Drawing for the job (mm, zero at the part's lowest x, y, z). A direction names the side the tool comes from. Coordinates: 2 decimals unless noted, no trailing zeros. Write each loop counter-clockwise with the first axis right and the second up, starting at its lowest first coordinate (ties: lowest second). Pieces come first, ordered by that corner, then holes. Notation, with made-up numbers: (22.25, 42) - (72.25, 42) arc R27 ccw to (72.25, 69) - close; hole circle Ø7 at (53, 27.5). An arc over 180 degrees is marked (long way). Write each question's results on one line, items separated by ' | '.
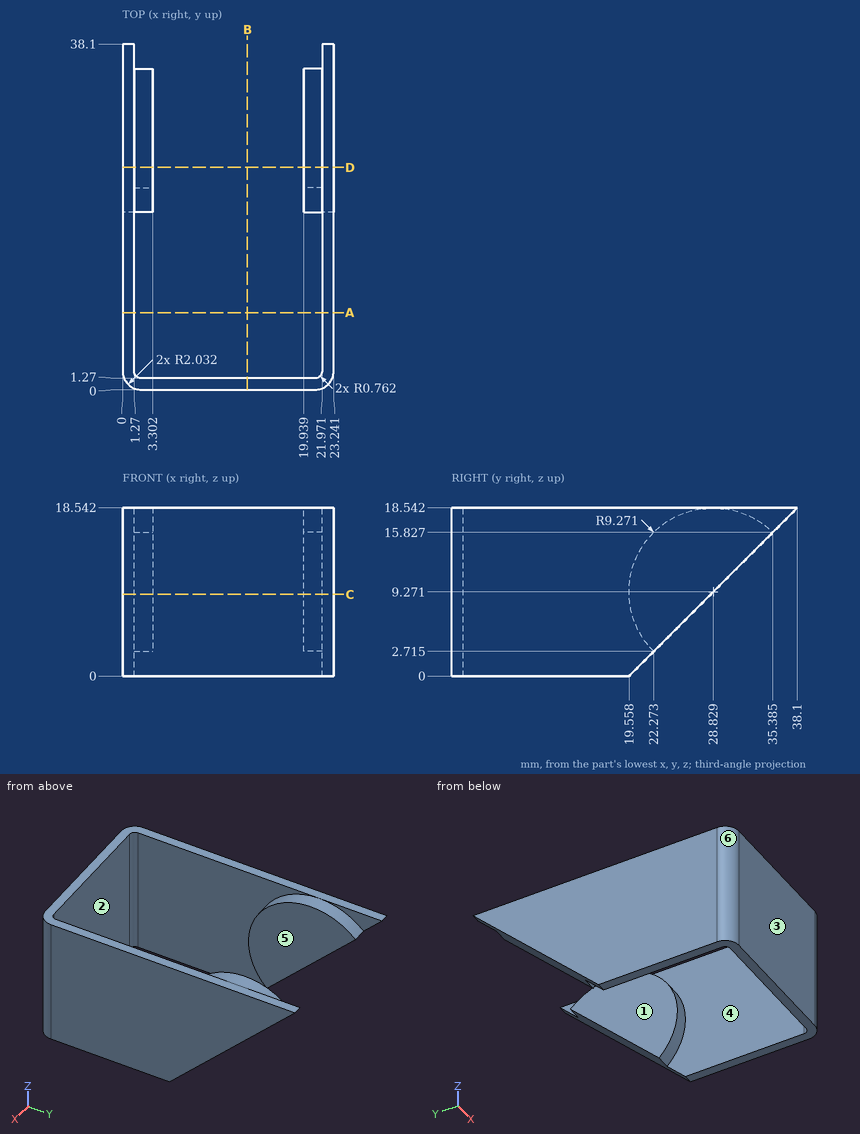
(1) Flat gauge pins, fed straight in: P1, Ø8, axis at y = 29.5, z = 9.5, coming from the +X side; P2, Ø1, axis at x = 20.5, y = 27.5, coming from the +Z side (1 decimal); P3, Ø8, axis at x = 13, z = 9, coming from the +Y side. Where does each tip first touch, or does it go through?
Return value:
P1: stops at x = 23.24 | P2: stops at z = 18.5 | P3: stops at y = 1.27
(2) Saw through at A-A on y = 8.5. Write the cut outline in (x, z).
Return value:
outline: (0, 0) - (1.27, 0) - (1.27, 18.54) - (0, 18.54) - close; (21.97, 0) - (23.24, 0) - (23.24, 18.54) - (21.97, 18.54) - close
(3) Saw through at B-B on x = 13.75. Write the cut outline in (y, z).
Return value:
outline: (0, 0) - (1.27, 0) - (1.27, 18.54) - (0, 18.54) - close
(4) Saw through at D-D on y = 24.5. Write the cut outline in (x, z).
Return value:
outline: (0, 4.94) - (3.3, 4.94) - (3.3, 17.47) - (1.27, 17.47) - (1.27, 18.54) - (0, 18.54) - close; (19.94, 4.94) - (23.24, 4.94) - (23.24, 18.54) - (21.97, 18.54) - (21.97, 17.47) - (19.94, 17.47) - close
(5) Wall check: line 1 (X direction, y = 5.5, z = 1.25); line 2 (X direction, y = 25, z = 15.5); line 3 (Y direction, x = 18.75, z = 1.5). Give the ranges that are in metal, low to high. Write a range as from..to.
Return value:
line 1: x = 0..1.27, 21.97..23.24 | line 2: x = 0..3.3, 19.94..23.24 | line 3: y = 0..1.27
(6) Saw through at C-C on z = 9. Write the cut outline in (x, y).
Return value:
outline: (0, 2.03) arc R2.03 ccw to (2.03, 0) - (21.21, 0) arc R2.03 ccw to (23.24, 2.03) - (23.24, 28.56) - (19.94, 28.56) - (19.94, 19.56) - (21.97, 19.56) - (21.97, 2.03) arc R0.76 cw to (21.21, 1.27) - (2.03, 1.27) arc R0.76 cw to (1.27, 2.03) - (1.27, 19.56) - (3.3, 19.56) - (3.3, 28.56) - (0, 28.56) - close
(7) 3-axis set-ups, long thin cutter, end or side, ignore diameter. For the marked faces 1, 2 and 3: which of +Z, -Z, +X, -X, +Y, -Y reach the whole face in a straight line?
Return value:
face 1: +Z, -Z, +Y | face 2: +Z, -Z | face 3: +Z, -Z, +X, -X, -Y
(8) Two-plate mould, pull along Y, no slides. Class the marked faces 4, 5 and 6: released by +Y, released by -Y, zero draft, split by the parting line, or undercut.
Return value:
face 4: undercut | face 5: zero draft | face 6: released by -Y
